For this review, take the finished solid that the model builds, in its own axes (mm). A direction names the side the tool comes from. Round coordinates to 2 decimals unless told otherwise and drop trailing zeros. Write each loop counter-clockwise with the first axis right and the second up, starting at its lowest first coordinate (ties: lowest second). Pieces come first, ordered by that corner, then holes. Notation, with made-up numbers: M -13.75,89 L 8.25,89 A20 cw 8.25,124 Z; hole C -9.5,-4.5 d4. An arc over 180 degrees is marked long. One line per question, with ' | ' between items.
```python
from build123d import *

# Parameters (mm, degrees)
SKETCH1_R                = 1.542
BOSS_EXTRUDE1_DEPTH      = 5
BOSS_EXTRUDE4_DEPTH      = 50
BOSS_EXTRUDE4_DEPTH_BACK = 5
FILLET3_R                = 3
FILLET4_R                = 5
BOSS_EXTRUDE5_DEPTH      = 55
SKETCH7_W                = 15
SKETCH7_H                = 25
BOSS_EXTRUDE6_DEPTH      = 36.5
SKETCH8_R                = 1
CUT_EXTRUDE1_DEPTH       = 88.266832187
SKETCH9_W                = 150
SKETCH9_H                = 30
BOSS_EXTRUDE7_DEPTH      = 5
FILLET5_R                = 3
FILLET6_R                = 3


with BuildPart() as part:
    # Sketch1 → Boss-Extrude1 (new body)
    with BuildSketch(Plane.XY):
        Polygon((-17.5, 17.5), (17.5, 17.5), (21.5, 17.5), (21.5, -21.5), (17.5, -21.5), (-17.5, -21.5), (-17.5, -17.5), align=None)
        with Locations((-12.078444483, 12.078444483)):
            Circle(SKETCH1_R, mode=Mode.SUBTRACT)
        with Locations(Location((12.078444483, 12.078444483, 0), (0, 0, 180))):
            Circle(SKETCH1_R, mode=Mode.SUBTRACT)
        with Locations((12.078444483, -12.078444483)):
            Circle(SKETCH1_R, mode=Mode.SUBTRACT)
        with Locations(Location((-12.078444483, -12.078444483, 0), (0, 0, 180))):
            Circle(SKETCH1_R, mode=Mode.SUBTRACT)
    extrude(amount=BOSS_EXTRUDE1_DEPTH)

    # Sketch4 → Boss-Extrude4 (add, two sides: drawn at the far end of the back side and taken through both)
    with BuildSketch(Plane.XY.offset(5).offset(-BOSS_EXTRUDE4_DEPTH_BACK)):
        Polygon((21.5, 17.5), (26, 17.5), (26, -26), (-17.5, -26), (-17.5, -21.5), (21.5, -21.5), align=None)
    extrude(amount=BOSS_EXTRUDE4_DEPTH + BOSS_EXTRUDE4_DEPTH_BACK)

    # Fillet3
    fillet3_edges = [part.edges().sort_by_distance(p)[0] for p in [
        (2, -21.5, 5),
        (21.5, -2, 5),
    ]]
    fillet(fillet3_edges, radius=FILLET3_R)

    # Fillet4
    # the kernel refuses this fillet: 5 mm, written as the material it adds along each edge
    with BuildSketch(Plane(origin=(16.5, -16.5, 5), x_dir=(1, 0, 0), z_dir=(0, 1, 0))) as fillet4_piece_1:
        with BuildLine():
            CenterArc((2, -3), 3, 0, 90)
            Line((5, -3), (5, 0))
            Line((5, 0), (2, 0))
        make_face()
    revolve(axis=Axis((16.5, -16.5, 5), (0, 0, -1)), revolution_arc=90)
    with BuildSketch(Plane(origin=(21.5, -21.5, 5), x_dir=(0, 1, 0), z_dir=(0, 0, 1))) as fillet4_piece_2:
        with BuildLine():
            CenterArc((FILLET4_R, FILLET4_R), FILLET4_R, 180, 90)
            Line((0, FILLET4_R), (0, 0))
            Line((0, 0), (FILLET4_R, 0))
        make_face()
    extrude(amount=50)

    # Sketch6 → Boss-Extrude5 (add, through all)
    with BuildSketch(Plane.XY.offset(55)):
        Polygon((-17.5, -26), (26, -26), (26, 17.5), (33, 17.5), (33, -39.5), (26, -39.5), (-17.5, -39.5), align=None)
    extrude(amount=-BOSS_EXTRUDE5_DEPTH)

    # Sketch7 → Boss-Extrude6 (add)
    with BuildSketch(Plane(origin=(33, 0, 0), x_dir=(0, 0, -1), z_dir=(1, 0, 0))):
        with Locations((-27.5, -11)):
            Rectangle(SKETCH7_W, SKETCH7_H)
    extrude(amount=BOSS_EXTRUDE6_DEPTH)

    # Sketch8 → Cut-Extrude1 (cut, through all)
    with BuildSketch(Plane.XY.offset(35)):
        with Locations((51.25, -11)):
            Circle(SKETCH8_R)
        with Locations((51.25, -16)):
            Circle(SKETCH8_R)
        with Locations((51.25, -6)):
            Circle(SKETCH8_R)
    extrude(amount=-CUT_EXTRUDE1_DEPTH, mode=Mode.SUBTRACT)

    # Sketch9 → Boss-Extrude7 (add)
    with BuildSketch(Plane(origin=(69.5, 0, 0), x_dir=(0, 0, -1), z_dir=(1, 0, 0))):
        with Locations((5, -11)):
            Rectangle(SKETCH9_W, SKETCH9_H)
    extrude(amount=-BOSS_EXTRUDE7_DEPTH)

    # Fillet5
    # the kernel refuses this fillet: 3 mm, written as the material it adds along each edge
    with BuildSketch(Plane(origin=(64.5, -23.5, 35), x_dir=(-1, 0, 0), z_dir=(0, 0, -1)), Plane(origin=(64.5, 1.5, 20), x_dir=(-1, 0, 0), z_dir=(0, 0, 1))) as fillet5_piece_1:
        with BuildLine():
            CenterArc((2.958039892, -3), FILLET5_R, 90, 80.405931773)
            Line((0, -2.5), (-0.059160798, -2.49))
            ThreePointArc((-0.059160798, -2.49), (-0.06, -1.25), (-0.06, 0))
            Line((-0.06, 0), (0, 0.06))
            Line((0, 0.06), (2.958039892, 0.06))
            Line((2.958039892, 0.06), (2.958039892, 0))
        make_face()
    extrude(amount=15)
    with BuildSketch(Plane(origin=(64.5, -23.5, 20), x_dir=(-1, 0, 0), z_dir=(0, 1, 0)), Plane(origin=(64.5, 1.5, 35), x_dir=(-1, 0, 0), z_dir=(0, -1, 0))) as fillet5_piece_2:
        with BuildLine():
            CenterArc((FILLET5_R, -FILLET5_R), FILLET5_R, 90, 90)
            Line((0, -FILLET5_R), (-FILLET5_R * 0.02, -FILLET5_R))
            Line((-FILLET5_R * 0.02, -FILLET5_R), (-FILLET5_R * 0.02, FILLET5_R * 0.02))
            Line((-FILLET5_R * 0.02, FILLET5_R * 0.02), (FILLET5_R, FILLET5_R * 0.02))
            Line((FILLET5_R, FILLET5_R * 0.02), (FILLET5_R, 0))
        make_face()
    extrude(amount=25)
    with BuildSketch(Plane(origin=(64.5, -23.5, 42.395099729), x_dir=(-1, 0, 0), z_dir=(0, 0, -1))) as fillet5_piece_3a_section:
        with BuildLine():
            CenterArc((2.958039892, -3), FILLET5_R, 90, 80.405931773)
            Line((0, -2.5), (-0.059160798, -2.49))
            ThreePointArc((-0.059160798, -2.49), (-0.06, -1.25), (-0.06, 0))
            Line((-0.06, 0), (0, 0.06))
            Line((0, 0.06), (2.958039892, 0.06))
            Line((2.958039892, 0.06), (2.958039892, 0))
        make_face()
    fillet5_piece_3a = extrude(amount=22.395099729, mode=Mode.PRIVATE)
    fillet5_piece_3a = split(fillet5_piece_3a, bisect_by=Plane(origin=(63.81401797, -24.116958935, 35), z_dir=(0, 0, 1)), keep=Keep.TOP, mode=Mode.PRIVATE)
    with BuildSketch(Plane(origin=(64.5, 1.5, 35), x_dir=(-1, 0, 0), z_dir=(0, -1, 0))) as fillet5_piece_3b_section:
        with BuildLine():
            CenterArc((FILLET5_R, -FILLET5_R), FILLET5_R, 90, 90)
            Line((0, -FILLET5_R), (-FILLET5_R * 0.02, -FILLET5_R))
            Line((-FILLET5_R * 0.02, -FILLET5_R), (-FILLET5_R * 0.02, FILLET5_R * 0.02))
            Line((-FILLET5_R * 0.02, FILLET5_R * 0.02), (FILLET5_R, FILLET5_R * 0.02))
            Line((FILLET5_R, FILLET5_R * 0.02), (FILLET5_R, 0))
        make_face()
    fillet5_piece_3b = extrude(amount=32.5, mode=Mode.PRIVATE)
    fillet5_piece_3b = split(fillet5_piece_3b, bisect_by=Plane(origin=(63.820814657, -23.5, 35.679185343), z_dir=(0, -1, 0)), keep=Keep.TOP, mode=Mode.PRIVATE)
    fillet5_piece_3b = split(fillet5_piece_3b, bisect_by=Plane(origin=(63.820814657, -26, 35.679185343), z_dir=(0, 1, 0)), keep=Keep.TOP, mode=Mode.PRIVATE)
    fillet5_piece_3 = fillet5_piece_3a & fillet5_piece_3b
    add(fillet5_piece_3)
    with BuildSketch(Plane(origin=(64.5, -31, 20), x_dir=(-1, 0, 0), z_dir=(0, 1, 0))) as fillet5_piece_4a_section:
        with BuildLine():
            CenterArc((FILLET5_R, -FILLET5_R), FILLET5_R, 90, 90)
            Line((0, -FILLET5_R), (-FILLET5_R * 0.02, -FILLET5_R))
            Line((-FILLET5_R * 0.02, -FILLET5_R), (-FILLET5_R * 0.02, FILLET5_R * 0.02))
            Line((-FILLET5_R * 0.02, FILLET5_R * 0.02), (FILLET5_R, FILLET5_R * 0.02))
            Line((FILLET5_R, FILLET5_R * 0.02), (FILLET5_R, 0))
        make_face()
    fillet5_piece_4a = extrude(amount=32.5, mode=Mode.PRIVATE)
    fillet5_piece_4a = split(fillet5_piece_4a, bisect_by=Plane(origin=(63.820814657, -23.5, 19.320814657), z_dir=(0, -1, 0)), keep=Keep.TOP, mode=Mode.PRIVATE)
    fillet5_piece_4a = split(fillet5_piece_4a, bisect_by=Plane(origin=(63.820814657, -26, 19.320814657), z_dir=(0, 1, 0)), keep=Keep.TOP, mode=Mode.PRIVATE)
    with BuildSketch(Plane(origin=(64.5, -23.5, 35), x_dir=(-1, 0, 0), z_dir=(0, 0, -1))) as fillet5_piece_4b_section:
        with BuildLine():
            CenterArc((2.958039892, -3), FILLET5_R, 90, 80.405931773)
            Line((0, -2.5), (-0.059160798, -2.49))
            ThreePointArc((-0.059160798, -2.49), (-0.06, -1.25), (-0.06, 0))
            Line((-0.06, 0), (0, 0.06))
            Line((0, 0.06), (2.958039892, 0.06))
            Line((2.958039892, 0.06), (2.958039892, 0))
        make_face()
    fillet5_piece_4b = extrude(amount=22.395099729, mode=Mode.PRIVATE)
    fillet5_piece_4b = split(fillet5_piece_4b, bisect_by=Plane(origin=(63.81401797, -24.116958935, 20), z_dir=(0, 0, -1)), keep=Keep.TOP, mode=Mode.PRIVATE)
    fillet5_piece_4 = fillet5_piece_4a & fillet5_piece_4b
    add(fillet5_piece_4)
    with BuildSketch(Plane(origin=(64.5, 1.5, 12.604900271), x_dir=(-1, 0, 0), z_dir=(0, 0, 1))) as fillet5_piece_5a_section:
        with BuildLine():
            CenterArc((2.958039892, -3), FILLET5_R, 90, 80.405931773)
            Line((0, -2.5), (-0.059160798, -2.49))
            ThreePointArc((-0.059160798, -2.49), (-0.06, -1.25), (-0.06, 0))
            Line((-0.06, 0), (0, 0.06))
            Line((0, 0.06), (2.958039892, 0.06))
            Line((2.958039892, 0.06), (2.958039892, 0))
        make_face()
    fillet5_piece_5a = extrude(amount=22.395099729, mode=Mode.PRIVATE)
    fillet5_piece_5a = split(fillet5_piece_5a, bisect_by=Plane(origin=(63.81401797, 2.116958935, 20), z_dir=(0, 0, -1)), keep=Keep.TOP, mode=Mode.PRIVATE)
    with BuildSketch(Plane(origin=(64.5, -23.5, 20), x_dir=(-1, 0, 0), z_dir=(0, 1, 0))) as fillet5_piece_5b_section:
        with BuildLine():
            CenterArc((FILLET5_R, -FILLET5_R), FILLET5_R, 90, 90)
            Line((0, -FILLET5_R), (-FILLET5_R * 0.02, -FILLET5_R))
            Line((-FILLET5_R * 0.02, -FILLET5_R), (-FILLET5_R * 0.02, FILLET5_R * 0.02))
            Line((-FILLET5_R * 0.02, FILLET5_R * 0.02), (FILLET5_R, FILLET5_R * 0.02))
            Line((FILLET5_R, FILLET5_R * 0.02), (FILLET5_R, 0))
        make_face()
    fillet5_piece_5b = extrude(amount=32.5, mode=Mode.PRIVATE)
    fillet5_piece_5b = split(fillet5_piece_5b, bisect_by=Plane(origin=(63.820814657, 1.5, 19.320814657), z_dir=(0, 1, 0)), keep=Keep.TOP, mode=Mode.PRIVATE)
    fillet5_piece_5b = split(fillet5_piece_5b, bisect_by=Plane(origin=(63.820814657, 4, 19.320814657), z_dir=(0, -1, 0)), keep=Keep.TOP, mode=Mode.PRIVATE)
    fillet5_piece_5 = fillet5_piece_5a & fillet5_piece_5b
    add(fillet5_piece_5)
    with BuildSketch(Plane(origin=(64.5, 1.5, 20), x_dir=(-1, 0, 0), z_dir=(0, 0, 1))) as fillet5_piece_6a_section:
        with BuildLine():
            CenterArc((2.958039892, -3), FILLET5_R, 90, 80.405931773)
            Line((0, -2.5), (-0.059160798, -2.49))
            ThreePointArc((-0.059160798, -2.49), (-0.06, -1.25), (-0.06, 0))
            Line((-0.06, 0), (0, 0.06))
            Line((0, 0.06), (2.958039892, 0.06))
            Line((2.958039892, 0.06), (2.958039892, 0))
        make_face()
    fillet5_piece_6a = extrude(amount=22.395099729, mode=Mode.PRIVATE)
    fillet5_piece_6a = split(fillet5_piece_6a, bisect_by=Plane(origin=(63.81401797, 2.116958935, 35), z_dir=(0, 0, 1)), keep=Keep.TOP, mode=Mode.PRIVATE)
    with BuildSketch(Plane(origin=(64.5, 9, 35), x_dir=(-1, 0, 0), z_dir=(0, -1, 0))) as fillet5_piece_6b_section:
        with BuildLine():
            CenterArc((FILLET5_R, -FILLET5_R), FILLET5_R, 90, 90)
            Line((0, -FILLET5_R), (-FILLET5_R * 0.02, -FILLET5_R))
            Line((-FILLET5_R * 0.02, -FILLET5_R), (-FILLET5_R * 0.02, FILLET5_R * 0.02))
            Line((-FILLET5_R * 0.02, FILLET5_R * 0.02), (FILLET5_R, FILLET5_R * 0.02))
            Line((FILLET5_R, FILLET5_R * 0.02), (FILLET5_R, 0))
        make_face()
    fillet5_piece_6b = extrude(amount=32.5, mode=Mode.PRIVATE)
    fillet5_piece_6b = split(fillet5_piece_6b, bisect_by=Plane(origin=(63.820814657, 1.5, 35.679185343), z_dir=(0, 1, 0)), keep=Keep.TOP, mode=Mode.PRIVATE)
    fillet5_piece_6b = split(fillet5_piece_6b, bisect_by=Plane(origin=(63.820814657, 4, 35.679185343), z_dir=(0, -1, 0)), keep=Keep.TOP, mode=Mode.PRIVATE)
    fillet5_piece_6 = fillet5_piece_6a & fillet5_piece_6b
    add(fillet5_piece_6)

    # Fillet6
    fillet6_edges = [part.edges().sort_by_distance(p)[0] for p in [
        (33, -11, 20),
        (33, 1.5, 27.5),
        (33, -11, 35),
        (33, -23.5, 27.5),
    ]]
    fillet(fillet6_edges, radius=FILLET6_R)


solid = part.part
```
Item 1: Take a section at A-A (z = 1.5). Write out the cut boundary in (x, y).
Results:
outline: M -17.5,-39.5 L 33,-39.5 L 33,17.5 L -17.5,17.5 Z; M 64.5,-26 L 69.5,-26 L 69.5,4 L 64.5,4 Z; hole C -12.08,-12.08 d3.08; hole C -12.08,12.08 d3.08; hole C 12.08,-12.08 d3.08; hole C 12.08,12.08 d3.08
Item 2: Take a section at C-C (y = 7). Write out the cut boundary in (x, z).
Results:
outline: M -17.5,0 L 33,0 L 33,55 L 21.5,55 L 21.5,8 A3 cw 18.5,5 L -17.5,5 Z
Item 3: Insertion check: pin 1 Ø4 at (y, z) = (4.5, 17) entering from -X; pin 2 Ø5.5 at (x, z) = (67, 3) entering from -Y; pin 3 Ø12 at (x, y) = (50.5, -6) entering from -Z. Each pin has a flat end and moves straight along its axis. Give the tip position at first contact, or say it passes through.
Results:
pin 1: x = 21.5 | pin 2: y = -26 | pin 3: z = 20
Item 4: To check wall thickness, follow line 1 along Y through (x, z) = (51.25, 29.75); line 2 along X through (y, z) = (-4.5, 48); line 3 along X through (y, z) = (-5, -60). State the ranges of each line that lie inside material, in increasing order. Write a range as from..to.
Results:
line 1: -23.5..-17, -15..-12, -10..-7, -5..1.5 | line 2: 21.5..33, 64.5..69.5 | line 3: 64.5..69.5
Item 5: Take a section at B-B (x = 7.5). Write out the cut boundary in (y, z).
Results:
outline: M -39.5,0 L 17.5,0 L 17.5,5 L -18.5,5 A3 cw -21.5,8 L -21.5,55 L -39.5,55 Z
Item 6: Take a section at D-D (z = -39). Write out the cut boundary in (x, y), then the cut area to 3 significant figures.
Results:
outline: M 64.5,-26 L 69.5,-26 L 69.5,4 L 64.5,4 Z | area: 150 mm2
Item 7: Machinability: for faces 1 (the face through (63.456, 2.19, 27.353)), 2 (the face through (33.9, -24.36, 27.35)), 3 (the face through (33.9, -10.78, 19.14)), which of the approach directions +Z, -Z, +X, -X, +Y, -Y give a long, thin tool a straight path to every point of the face, cutting with its end or side? Answer none if there is none.
Results:
face 1: +Z, -Z, +Y | face 2: +Z, -Z, -Y | face 3: -Z, +Y, -Y
Item 8: Mouldability with a two-part tool opening along X and no side actions: class faces 4 (the face through (24, 17.5, 22)), 5 (the face through (69.5, -11, -4)), 6 (the face through (63.6, -11.21, 19.14)), 7 (the face through (20.6, 0.26, 5.86)) as +X half, -X half, draft (parallel to the pull), parting line (faces both ways), or undercut.
Results:
face 4: draft | face 5: +X half | face 6: undercut | face 7: -X half
